Geometry: final body of the model. Coordinates: model frame, mm. A direction names the side the tool comes from. Coordinates: 2 decimals unless noted, no trailing zeros. Write each loop counter-clockwise with the first axis right and the second up, starting at its lowest first coordinate (ties: lowest second). Pieces come first, ordered by that corner, then holes. Notation, with made-up numbers: (21.25, -8) - (63.25, -8) arc R26 ccw to (63.25, 18) - close; hole circle Ø3 at (31.5, 38). An arc over 180 degrees is marked (long way). Put each result on its own line as item: value.
```python
from build123d import *

# Parameters (mm, degrees)
BOSS_EXTRUDE1_DEPTH = 4.3
FILLET1_R           = 10


with BuildPart() as part:
    # Sketch1 → Boss-Extrude1 (new body)
    with BuildSketch(Plane(origin=(0, 0, 0), x_dir=(1, 0, 0), z_dir=(0, 1, 0))):
        Polygon((0, 0), (0, 80), (12, 80), (12, 73), (22, 73), (22, 80), (34, 80), (34, 73), (44, 73), (44, 80), (56, 80), (56, 0), align=None)
        with BuildLine():
            Line((14.966953147, 35), (14.966953147, 5))
            ThreePointArc((14.966953147, 5), (13, 3.033046853), (11.033046853, 5))
            Line((11.033046853, 5), (11.033046853, 35))
            ThreePointArc((11.033046853, 35), (13, 36.966953147), (14.966953147, 35))
        make_face(mode=Mode.SUBTRACT)
        with BuildLine():
            Line((8.5, 65), (8.5, 40))
            ThreePointArc((8.5, 40), (6, 37.5), (3.5, 40))
            Line((3.5, 40), (3.5, 65))
            ThreePointArc((3.5, 65), (6, 67.5), (8.5, 65))
        make_face(mode=Mode.SUBTRACT)
        with BuildLine():
            Line((41.033046853, 35), (41.033046853, 5))
            ThreePointArc((41.033046853, 5), (43, 3.033046853), (44.966953147, 5))
            Line((44.966953147, 5), (44.966953147, 35))
            ThreePointArc((44.966953147, 35), (43, 36.966953147), (41.033046853, 35))
        make_face(mode=Mode.SUBTRACT)
        with BuildLine():
            Line((25.5, 65), (25.5, 40))
            ThreePointArc((25.5, 40), (28, 37.5), (30.5, 40))
            Line((30.5, 40), (30.5, 65))
            ThreePointArc((30.5, 65), (28, 67.5), (25.5, 65))
        make_face(mode=Mode.SUBTRACT)
        with BuildLine():
            Line((47.5, 65), (47.5, 40))
            ThreePointArc((47.5, 40), (50, 37.5), (52.5, 40))
            Line((52.5, 40), (52.5, 65))
            ThreePointArc((52.5, 65), (50, 67.5), (47.5, 65))
        make_face(mode=Mode.SUBTRACT)
    extrude(amount=BOSS_EXTRUDE1_DEPTH)

    # Fillet1
    fillet1_edges = [part.edges().sort_by_distance(p)[0] for p in [
        (0, 2.15, 0),
        (56, 2.15, 0),
    ]]
    fillet(fillet1_edges, radius=FILLET1_R)


solid = part.part
```
1. Pin query (flat end, axial travel): pin 1 Ø1.3 at (x, y) = (17, 3) entering from -Z. Return the tip coordinate at first contact, or that it passes through.
Answer below:
pin 1: stops at z = -73
2. Set-up query: faces 1 (the flat face through (22, 2, -76)), 2 (the cylindrical face through (28.1, 2.1, -67.5)), 3 (the flat face through (28, 2, 0)). Return all of +Z, -Z, +X, -X, +Y, -Y with unobstructed straight access to the full face (end or side cutting, diameter ignored); none if empty.
Answer below:
face 1: -Z, +Y, -Y
face 2: +Y, -Y
face 3: +Z, +X, -X, +Y, -Y
3. Section query D-D (y = 2.2). Count the separate pieces of the cut face and the enclosed holes in it, then the cut area to 3 significant figures.
Answer below:
separate pieces: 1
enclosed holes: 5
area: 3,600 mm²
4. Section query B-B (x = 43). Return loops of the section in (y, z).
Answer below:
outline: (0, -73) - (4.3, -73) - (4.3, -36.97) - (0, -36.97) - close; (0, -3.03) - (4.3, -3.03) - (4.3, 0) - (0, 0) - close
5. Section query C-C (z = -50.5). Return loops of the section in (x, y).
Answer below:
outline: (0, 0) - (3.5, 0) - (3.5, 4.3) - (0, 4.3) - close; (8.5, 0) - (25.5, 0) - (25.5, 4.3) - (8.5, 4.3) - close; (30.5, 0) - (47.5, 0) - (47.5, 4.3) - (30.5, 4.3) - close; (52.5, 0) - (56, 0) - (56, 4.3) - (52.5, 4.3) - close
6. Mould query, pull axis Z, two halves, no side actions, for faces 4 (the flat face through (34, 2, -77)), 5 (the flat face through (44.967, 2, -20)), 6 (the cylindrical face through (2.85, 2.18, -3.01)). Classes: +Z half, -Z half, draft (parallel to the pull), parting line (faces both ways), or undercut.
Answer below:
face 4: draft
face 5: undercut
face 6: +Z half
7. Section query A-A (z = -26). Return loops of the section in (x, y), then the cut area to 3 significant figures.
Answer below:
outline: (0, 0) - (11.03, 0) - (11.03, 4.3) - (0, 4.3) - close; (14.97, 0) - (41.03, 0) - (41.03, 4.3) - (14.97, 4.3) - close; (44.97, 0) - (56, 0) - (56, 4.3) - (44.97, 4.3) - close
area: 207 mm²
8. Ray query, probe 1 along X at (y, z) = (3.2, -43); probe 2 along X at (y, z) = (3.4, -18); probe 3 along X at (y, z) = (3.05, -38.5). Return the intervals inside material, ascending. Write a range as from..to.
Answer below:
probe 1: x = 0..3.5, 8.5..25.5, 30.5..47.5, 52.5..56
probe 2: x = 0..11.03, 14.97..41.03, 44.97..56
probe 3: x = 0..4, 8..26, 30..48, 52..56
